```python
from build123d import *

# Parameters (mm, degrees)
SKETCH1_R           = 13
BOSS_EXTRUDE1_DEPTH = 30
SKETCH2_R           = 5
BOSS_EXTRUDE2_DEPTH = 240
SKETCH3_R           = 5
BOSS_EXTRUDE3_DEPTH = 20
FILLET1_R           = 2


with BuildPart() as part:
    # Sketch1 → Boss-Extrude1 (new body)
    with BuildSketch(Plane.XY):
        Circle(SKETCH1_R)
    extrude(amount=-BOSS_EXTRUDE1_DEPTH)

    # Sketch2 → Boss-Extrude2 (add)
    with BuildSketch(Plane.XY):
        Circle(SKETCH2_R)
    extrude(amount=BOSS_EXTRUDE2_DEPTH)

    # Sketch3 → Boss-Extrude3 (add)
    with BuildSketch(Plane.XY.offset(240)):
        Circle(SKETCH3_R)
    extrude(amount=BOSS_EXTRUDE3_DEPTH)

    # Fillet1
    fillet1_edges = [part.edges().sort_by_distance(p)[0] for p in [
        (-13, 0, 0),
        (-13, 0, -30),
        (-5, 0, 0),
    ]]
    fillet(fillet1_edges, radius=FILLET1_R)


solid = part.part
```
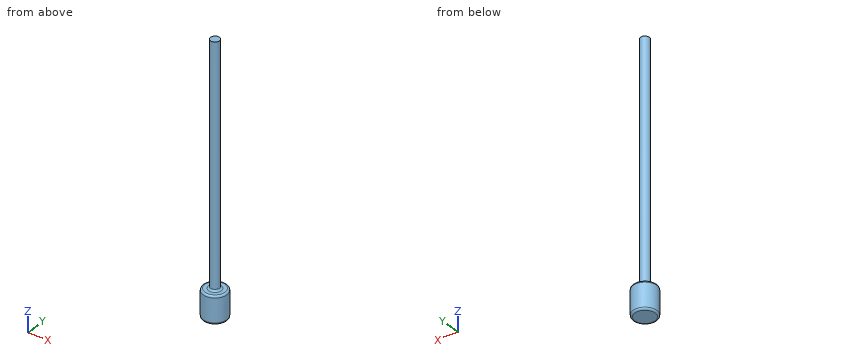
Could you check a few things on this model? Use its own coordinates, in mm. Give positions to 0.01 mm unless a question says otherwise; leave off trailing zeros. Order: outer loops, then holes, each group sorted by start corner. A loop starts at its lowest first (then second) coordinate and runs counter-clockwise, first axis right, second up.
Q1. Suppose I cut it at A-A, the plane y = 0. Write out the boundary of the cut face in (x, z), and give its area (3 significant figures).
Q2. Suppose I cut it at C-C, the plane z = 242. Write out the boundary of the cut face in (x, y).
Q3. I'm going to push flat-ended pins straight in: P1, Ø10, axis at x = 2, z = 58.5, coming from the -Y side; P2, Ø12, axis at y = -2.5, z = 204.5, coming from the +X side; P3, Ø1, axis at x = -5, z = 32.5, coming from the -Y side. Where does each tip first touch, or does it pass through?
Q4. If I drill on line 1 along Z through (x, y) = (3.75, -6.5); line 2 along Y through (x, z) = (-0.25, 246.5); line 3 along X through (y, z) = (-0.75, -3.5), over which ranges is the centre line in solid material (lowest first)?
Solution:
1. outline: (-13, -28) arc R2 ccw to (-11, -30) - (11, -30) arc R2 ccw to (13, -28) - (13, -2) arc R2 ccw to (11, 0) - (7, 0) arc R2 cw to (5, 2) - (5, 260) - (-5, 260) - (-5, 2) arc R2 cw to (-7, 0) - (-11, 0) arc R2 ccw to (-13, -2) - close
1. area: 3,380 mm2
2. outline: circle Ø10 at (0, 0)
3. P1: stops at y = -5
3. P2: stops at x = 5
3. P3: stops at y = -2.18
4. line 1: z = -30 to 0
4. line 2: y = -4.99 to 4.99
4. line 3: x = -12.98 to 12.98
